```python
from build123d import *

# Parameters (mm, degrees)
F0_R     = 0.4490128061
F0_W     = 10.16
F0_H     = 5.08
F3_DEPTH = 1.5875
F4_R     = 0.508


with BuildPart() as f3:
    # F0 (on Top) → F3 (new body)
    with BuildSketch(Plane.XY):
        Polygon((24.13, 0), (24.13, 13.97), (1.27, 13.97), (1.27, 0), (8.89, 0), (8.89, 2.54), (16.51, 2.54), (16.51, 0), align=None)
        with Locations((10.16, 5.08)):
            Circle(F0_R, mode=Mode.SUBTRACT)
        with Locations((12.7, 5.08)):
            Circle(F0_R, mode=Mode.SUBTRACT)
        with Locations((15.24, 5.08)):
            Circle(F0_R, mode=Mode.SUBTRACT)
        with Locations((5.08, 10.16)):
            Circle(F0_R, mode=Mode.SUBTRACT)
        with Locations((13.97, 8.89)):
            Rectangle(F0_W, F0_H, mode=Mode.SUBTRACT)
        with Locations((20.32, 10.16)):
            Circle(F0_R, mode=Mode.SUBTRACT)
    extrude(amount=F3_DEPTH)

    # F4
    f4_edges = [f3.edges().sort_by_distance(p)[0] for p in [
        (1.27, 0, 0.79375),
        (8.89, 0, 0.79375),
        (16.51, 2.54, 0.79375),
        (16.51, 0, 0.79375),
        (24.13, 0, 0.79375),
        (8.89, 11.43, 0.79375),
        (8.89, 2.54, 0.79375),
        (24.13, 13.97, 0.79375),
        (8.89, 6.35, 0.79375),
        (1.27, 13.97, 0.79375),
        (19.05, 6.35, 0.79375),
        (19.05, 11.43, 0.79375),
    ]]
    fillet(f4_edges, radius=F4_R)


solid = f3.part
```
Verification items for the finished model (mm, model axes). A direction names the side the tool comes from. Coordinates: 2 decimals unless noted, no trailing zeros. Order: outer loops, then holes, each group sorted by start corner. A loop starts at its lowest first (then second) coordinate and runs counter-clockwise, first axis right, second up. Notation, with made-up numbers: (-14.75, 69) -> (38.25, 69) arc R19 cw to (38.25, 93) -> close; hole circle Ø2 at (80, 57.25). An arc over 180 degrees is marked (long way). Answer as CSV lines item,"result". Start each with the question number.
1) Set-up check for faces 1 (the face through (13, 13.97, 1)), 2 (the face through (8.89, 9, 1)), 3 (the face through (8.89, 1, 1)): record each of +Z, -Z, +X, -X, +Y, -Y from which the full face is reachable in a straight line by a thin tool's end or side.
2) Cross-section at C-C, the plane y = 5.08. Record the boundary of the cut face in (x, z), then the cut area to 3 significant figures.
3) Cross-section at D-D, the plane x = 20.32. Record the boundary of the cut face in (y, z).
4) Material ranges on L1, parallel to Y at x = 12.75, z = 0.5; L2, parallel to X at y = 7.25, z = 0.65; L3, parallel to Y at x = 10, z = 0.45, recorded low to high. Write a range as [from, to].
5) Cross-section at A-A, the plane x = 12.7. Record the boundary of the cut face in (y, z), then the cut area to 4 significant figures.
6) Release check for a two-part mould opening along Y. For faces 4 (the face through (13, 6, 0)), 5 (the face through (12.34, 4.81, 0.78)), 6 (the face through (20, 0, 1)) record: released by +Y, released by -Y, zero draft, split by the parting line, or undercut.
7) Cross-section at B-B, the plane z = 1.3. Give the number of separate pieces and of enclosed holes in the cut face, then the cut area to 3 significant figures.
Conclusion:
1,face 1,"+Z, -Z, +X, -X, +Y"
1,face 2,"+Z, -Z"
1,face 3,"+Z, -Z, -Y"
2,outline,"(1.27, 0) -> (9.71, 0) -> (9.71, 1.59) -> (1.27, 1.59) -> close; (10.61, 0) -> (12.25, 0) -> (12.25, 1.59) -> (10.61, 1.59) -> close; (13.15, 0) -> (14.79, 0) -> (14.79, 1.59) -> (13.15, 1.59) -> close; (15.69, 0) -> (24.13, 0) -> (24.13, 1.59) -> (15.69, 1.59) -> close"
2,area,"32.0 mm²"
3,outline,"(0, 0) -> (9.71, 0) -> (9.71, 1.59) -> (0, 1.59) -> close; (10.61, 0) -> (13.97, 0) -> (13.97, 1.59) -> (10.61, 1.59) -> close"
4,L1,"y = [2.54, 4.63], [5.53, 6.35], [11.43, 13.97]"
4,L2,"x = [1.27, 8.89], [19.05, 24.13]"
4,L3,"y = [2.54, 4.66], [5.5, 6.35], [11.43, 13.97]"
5,outline,"(2.54, 0) -> (4.63, 0) -> (4.63, 1.59) -> (2.54, 1.59) -> close; (5.53, 0) -> (6.35, 0) -> (6.35, 1.59) -> (5.53, 1.59) -> close; (11.43, 0) -> (13.97, 0) -> (13.97, 1.59) -> (11.43, 1.59) -> close"
5,area,"8.655 mm²"
6,face 4,"zero draft"
6,face 5,"undercut"
6,face 6,"released by -Y"
7,separate pieces,"1"
7,enclosed holes,"6"
7,area,"245 mm²"
